Work out the finished part from the listing and answer in its coordinate system (mm). A direction names the side the tool comes from. Coordinates: 2 decimals unless noted, no trailing zeros. Write each loop counter-clockwise with the first axis right and the second up, starting at its lowest first coordinate (ties: lowest second). Pieces come first, ordered by that corner, then holes. Notation, with made-up numbers: (-3, -14.75) - (7, -14.75) arc R24 ccw to (7, 15.25) - close; hole circle Ø5 at (75.5, 60). An arc over 180 degrees is marked (long way). Use CSV: the item, a comma, the result in double quotes. Start each with the question number.
from build123d import *

# Parameters (mm, degrees)
F0_R     = 3
F1_DEPTH = 4.2
F2_T     = -0.45
F3_DEPTH = 0.6


with BuildPart() as f1:
    # F0 (on Top) → F1 (new body)
    with BuildSketch(Plane.XY):
        Polygon((0, -6.2931179342), (5.45, -3.1465589671), (5.45, 3.1465589671), (0, 6.2931179342), (-5.45, 3.1465589671), (-5.45, -3.1465589671), align=None)
        Circle(F0_R, mode=Mode.SUBTRACT)
        Circle(F0_R)
    extrude(amount=F1_DEPTH)

    # F2
    f2_openings = [f1.faces().sort_by_distance(p)[0] for p in [
        (0, 0, 4.2),
    ]]
    offset(amount=F2_T, openings=f2_openings)

    # F0 (on Top) → F3 (cut)
    with BuildSketch(Plane.XY):
        Circle(F0_R)
    extrude(amount=F3_DEPTH, mode=Mode.SUBTRACT)


solid = f1.part
Item 1: Straight lines are drawn through the part: probe 1 along X at (y, z) = (-1, 2.85); probe 2 along X at (y, z) = (0, 0.2); probe 3 along Z at (x, y) = (-4.5, -0.25). For each, find the intervals that lie inside material, in ascending order. Write a range as [from, to].
Item 2: A cutting plane is placed at B-B (x = -1.5). Determine the outline of the cut face in (y, z), then the cut area to 3 significant figures.
Item 3: A cutting plane is placed at C-C (z = 1.75). Determine the outline of the cut face in (x, y), then the cut area to 3 significant figures.
Item 4: A cutting plane is placed at A-A (y = 0). Determine the outline of the cut face in (x, z), then the cut area to 3 significant figures.
Item 5: A cutting plane is placed at D-D (y = -3.5). Determine the outline of the cut face in (x, z).
Item 6: Determine the mould class of faces 1 (the face through (-2.69, 4.74, 2.07)), 2 (the face through (2.69, -4.74, 2.07)), 3 (the face through (-3, 0.1, 0.2)) for opening direction X: +X half, -X half, draft (parallel to the pull), parting line (faces both ways), or undercut.
Item 7: Which of the six approach directions +Z, -Z, +X, -X, +Y, -Y give full straight-line access (tool end or side, diameter ignored) to faces 4 (the face through (2.535, 4.31, 2.299)), 5 (the face through (-5.45, 0, 2))?
Item 8: This flat-tipped pin is pushed along its axis until it touches: pin 1 (1.5 mm diameter, centred on x = -0.5, y = 2.5, fed in from +Z). Where does it stop, or does it pass through?
Calculated:
1,probe 1,"x = [-5.45, -5], [5, 5.45]"
1,probe 2,"x = [-5.45, -3], [3, 5.45]"
1,probe 3,"z = [0, 0.45]"
2,outline,"(-5.43, 0) - (-2.6, 0) - (-2.6, 0.45) - (-4.91, 0.45) - (-4.91, 4.2) - (-5.43, 4.2) - close; (2.6, 0) - (5.43, 0) - (5.43, 4.2) - (4.91, 4.2) - (4.91, 0.45) - (2.6, 0.45) - close"
2,area,"6.44 mm²"
3,outline,"(-5.45, -3.15) - (0, -6.29) - (5.45, -3.15) - (5.45, 3.15) - (0, 6.29) - (-5.45, 3.15) - close; hole (-5, -2.89) - (0, -5.77) - (5, -2.89) - (5, 2.89) - (0, 5.77) - (-5, 2.89) - close"
3,area,"16.3 mm²"
4,outline,"(-5.45, 0) - (-3, 0) - (-3, 0.45) - (-5, 0.45) - (-5, 4.2) - (-5.45, 4.2) - close; (3, 0) - (5.45, 0) - (5.45, 4.2) - (5, 4.2) - (5, 0.45) - (3, 0.45) - close"
4,area,"5.58 mm²"
5,outline,"(-4.84, 0) - (4.84, 0) - (4.84, 4.2) - (3.94, 4.2) - (3.94, 0.45) - (-3.94, 0.45) - (-3.94, 4.2) - (-4.84, 4.2) - close"
6,face 1,"-X half"
6,face 2,"+X half"
6,face 3,"undercut"
7,face 4,"+Z"
7,face 5,"+Z, -Z, -X, +Y, -Y"
8,pin 1,"stops at z = 0.45"
